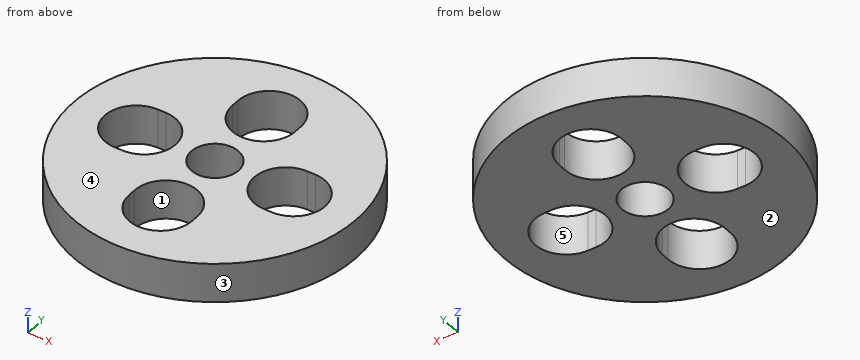
```python
from build123d import *

# Parameters (mm, degrees)
ESQUISSE1_R             = 18
ESQUISSE1_R_2           = 3.0025
BOSS_EXTRU_1_DEPTH      = 5
ENL_V_MAT_EXTRU_1_DEPTH = 5


with BuildPart() as part:
    # Esquisse1 → Boss.-Extru.1 (new body)
    with BuildSketch(Plane.XY):
        Circle(ESQUISSE1_R)
        Circle(ESQUISSE1_R_2, mode=Mode.SUBTRACT)
    extrude(amount=BOSS_EXTRU_1_DEPTH)

    # Esquisse2 → Enlèv. mat.-Extru.1 (cut)
    with BuildSketch(Plane.XY.offset(5)):
        with BuildLine():
            Line((-4, 10), (-4, 9))
            ThreePointArc((-4, 9), (0, 5), (4, 9))
            Line((4, 9), (4, 10))
            ThreePointArc((4, 10), (0, 14), (-4, 10))
        make_face()
        with BuildLine():
            Line((-10, -4), (-9, -4))
            ThreePointArc((-9, -4), (-5, 0), (-9, 4))
            Line((-9, 4), (-10, 4))
            ThreePointArc((-10, 4), (-14, 0), (-10, -4))
        make_face()
        with BuildLine():
            Line((4, -10), (4, -9))
            ThreePointArc((4, -9), (0, -5), (-4, -9))
            Line((-4, -9), (-4, -10))
            ThreePointArc((-4, -10), (0, -14), (4, -10))
        make_face()
        with BuildLine():
            Line((10, 4), (9, 4))
            ThreePointArc((9, 4), (5, 0), (9, -4))
            Line((9, -4), (10, -4))
            ThreePointArc((10, -4), (14, 0), (10, 4))
        make_face()
    extrude(amount=-ENL_V_MAT_EXTRU_1_DEPTH, mode=Mode.SUBTRACT)


solid = part.part
```
Check sheet for the modelled part. Datum: model origin and axes. Units: mm. Face numbers are marked on the shaded views. A direction names the side the tool comes from. Give positions to 0.01 mm unless a question says otherwise; leave off trailing zeros. Loops run counter-clockwise (first coordinate to the right, second up) from the corner with the lowest first, then second, coordinate; pieces in that order, holes last. Notation, with made-up numbers: M 17.25,-22 L 41.25,-22 A12 ccw 41.25,-15 Z; hole C -17.5,-12.75 d6. An arc over 180 degrees is marked long. Answer in a Markdown table with one row per item.
1) Depth check by flat-ended pin: pin 1 (1.5 mm diameter, centred on x = 4.5, z = 3.5, fed in from -Y); pin 2 (1 mm diameter, centred on x = 7.5, y = 6, fed in from -Z); pin 3 (0.8 mm diameter, centred on y = 9.5, z = 2.5, fed in from -X); pin 4 (0.5 mm diameter, centred on x = 9.5, z = 3, fed in from +Y). Enter the tip coordinate at first touch or a pass-through.
Solutions:
| item | result |
|---|---|
| pin 1 | stops at y = -17.61 |
| pin 2 | stops at z = 0 |
| pin 3 | stops at x = -15.53 |
| pin 4 | stops at y = 15.44 |
2) Thickness scan on line 1 (Y direction, x = 0, z = 4); line 2 (X direction, y = -10.5, z = 2); line 3 (X direction, y = 10, z = 1.2). Record the ranges inside material, lowest first.
Solutions:
| item | result |
|---|---|
| line 1 | y = -18 to -14, -5 to -3, 3 to 5, 14 to 18 |
| line 2 | x = -14.62 to -3.97, 3.97 to 14.62 |
| line 3 | x = -14.97 to -4, 4 to 14.97 |
3) Cross-section at C-C (y = -6). Enter the section's corners in (x, z), plus the area to 3 significant figures.
Solutions:
| item | result |
|---|---|
| outline | M -16.97,0 L -2.65,0 L -2.65,5 L -16.97,5 Z; M 2.65,0 L 16.97,0 L 16.97,5 L 2.65,5 Z |
| area | 143 mm^2 |
4) Cross-section at B-B (z = 3.95). Enter the section's corners in (x, y) (1 decimal).
Solutions:
| item | result |
|---|---|
| outline | C 0,0 d36; hole M -10,-4 L -9,-4 A4 ccw -9,4 L -10,4 A4 ccw Z; hole M -4,-10 A4 ccw 4,-10 L 4,-9 A4 ccw -4,-9 Z; hole M -4,9 A4 ccw 4,9 L 4,10 A4 ccw -4,10 Z; hole C 0,0 d6; hole M 9,-4 L 10,-4 A4 ccw 10,4 L 9,4 A4 ccw Z |
5) Mould release check, pull along X, two halves, no side actions. Record for the marked faces 1, 2 and 3: released by +X, released by -X, zero draft, split by the parting line, or undercut.
Solutions:
| item | result |
|---|---|
| face 1 | undercut |
| face 2 | zero draft |
| face 3 | split by the parting line |
6) Tool access check on the marked faces 4 and 5. Record the directions out of +Z, -Z, +X, -X, +Y, -Y that give a thin tool (end or side, any length) a straight path to the whole face; none if there is none.
Solutions:
| item | result |
|---|---|
| face 4 | +Z, +X, -X, +Y, -Y |
| face 5 | +Z, -Z |
7) Cross-section at D-D (x = 13.5). Enter the section's corners in (y, z).
Solutions:
| item | result |
|---|---|
| outline | M -11.91,0 L -1.94,0 L -1.94,5 L -11.91,5 Z; M 1.94,0 L 11.91,0 L 11.91,5 L 1.94,5 Z |
8) Cross-section at A-A (y = 0). Enter the section's corners in (x, z).
Solutions:
| item | result |
|---|---|
| outline | M -18,0 L -14,0 L -14,5 L -18,5 Z; M -5,0 L -3,0 L -3,5 L -5,5 Z; M 3,0 L 5,0 L 5,5 L 3,5 Z; M 14,0 L 18,0 L 18,5 L 14,5 Z |
